from build123d import *

# Parameters (mm, degrees)
SKETCH2_R           = 3.175
BOSS_EXTRUDE2_DEPTH = 5.207


with BuildPart() as part:
    # Sketch2 → Boss-Extrude2 (new body)
    with BuildSketch(Plane.XY):
        with BuildLine():
            Line((0, 0), (177.8, 0))
            Line((177.8, 0), (177.8, 25.4))
            Line((177.8, 25.4), (0, 25.4))
            ThreePointArc((0, 25.4), (-12.7, 12.7), (0, 0))
        make_face()
        with Locations((0, 12.7)):
            Circle(SKETCH2_R, mode=Mode.SUBTRACT)
        with Locations((50.8, 12.7)):
            Circle(SKETCH2_R, mode=Mode.SUBTRACT)
    extrude(amount=BOSS_EXTRUDE2_DEPTH)


solid = part.part
Source: CAD feature listing. Evaluate the final solid. Frame: model axes, mm. Give positions to 0.01 mm unless a question says otherwise; leave off trailing zeros. Write each loop counter-clockwise with the first axis right and the second up, starting at its lowest first coordinate (ties: lowest second). Pieces come first, ordered by that corner, then holes. Notation, with made-up numbers: M 27,0 L 33,0 A17 ccw 33,14 Z; hole C 59.5,77 d4. An arc over 180 degrees is marked long. Answer as a JSON object with one key per item and string values.
Q1. Cut plane C-C, the plane z = 1.9. Return the cut outline in (x, y) (3 decimals).
Geometry check:
{"outline": "M 0,0 L 177.8,0 L 177.8,25.4 L 0,25.4 A12.7 ccw Z; hole C 0,12.7 d6.35; hole C 50.8,12.7 d6.35"}
Q2. Cut plane A-A, the plane x = 50.8. Return the cut outline in (y, z) (3 decimals), then the cut area to 3 significant figures.
Geometry check:
{"outline": "M 0,0 L 9.525,0 L 9.525,5.207 L 0,5.207 Z; M 15.875,0 L 25.4,0 L 25.4,5.207 L 15.875,5.207 Z", "area": "99.2 mm^2"}
Q3. Mould query, pull axis Y, two halves, no side actions, for faces 1 (the face through (1.5, 9.9, 2.6)), 2 (the face through (-12.697, 12.979, 2.567)), 3 (the face through (88, 0, 3)). Classes: +Y half, -Y half, draft (parallel to the pull), parting line (faces both ways), or undercut.
Geometry check:
{"face 1": "undercut", "face 2": "parting line", "face 3": "-Y half"}
Q4. Cut plane B-B, the plane y = 12.7. Return the cut outline in (x, z) (3 decimals).
Geometry check:
{"outline": "M -12.7,0 L -3.175,0 L -3.175,5.207 L -12.7,5.207 Z; M 3.175,0 L 47.625,0 L 47.625,5.207 L 3.175,5.207 Z; M 53.975,0 L 177.8,0 L 177.8,5.207 L 53.975,5.207 Z"}
Q5. Cut plane D-D, the plane y = 3. Return the cut outline in (x, z), then the cut area to 3 significant figures.
Geometry check:
{"outline": "M -8.2,0 L 177.8,0 L 177.8,5.21 L -8.2,5.21 Z", "area": "968 mm^2"}
Q6. Contact query for a flat-ended pin moving along its axis: P1, Ø5.5, axis at x = 0, y = 12.7, coming from the +Z side. Output: stop coordinate, or through.
Geometry check:
{"P1": "passes through"}
Q7. Ray query, line 1 along Y through (x, z) = (0, 2.3) (3 decimals); line 2 along X through (y, z) = (12, 3.9); line 3 along X through (y, z) = (11, 3.3). Return the intervals inside material, ascending.
Geometry check:
{"line 1": "y = 0 to 9.525, 15.875 to 25.4", "line 2": "x = -12.68 to -3.1, 3.1 to 47.7, 53.9 to 177.8", "line 3": "x = -12.59 to -2.68, 2.68 to 48.12, 53.48 to 177.8"}
